Autodesk Inventor part; units mm, degrees
ref_plane "YZ Plane" through (0, 0, 0) normal (1, 0, 0) x (0, 1, 0)
ref_plane "XZ Plane" through (0, 0, 0) normal (0, 1, 0) x (-1, 0, 0)
ref_plane "XY Plane" through (0, 0, 0) normal (0, 0, 1) x (1, 0, 0)
sketch "スケッチ1" plane through (0, 0, 0) normal (0, 0, 1) x (1, 0, 0)
  circle A0 centre (0, 0) radius 7.5
  circle A1 centre (0, 0) radius 2
  dimension "d0" = 15
  dimension "d1" = 4
extrude "押し出し1" add sketch "スケッチ1" along normal blind 10 contours A1
extrude "押し出し2" add sketch "スケッチ1" against normal blind 15 contours A0 | A1
sketch "スケッチ2" plane through (0, 0, -15) normal (0, 0, -1) x (-1, 0, 0)
  circle A0 centre (0, 0) radius 7.5
hole "穴1" at (0, 0, -15) direction (0, 0, 1) diameter 3.3 depth 4 tip angle 118
properties part number "防振ゴム雄ねじ雌ねじm4スペーサー長さ15"
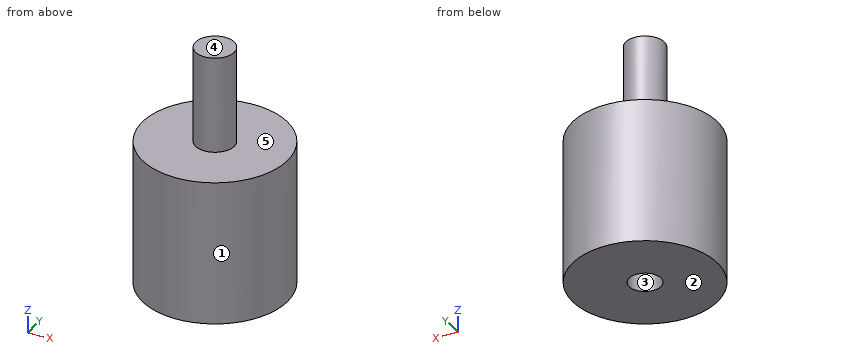
Work out the finished part from the listing and answer in its coordinate system (mm). Face numbers are marked on the shaded views. A direction names the side the tool comes from. Give positions to 0.01 mm unless a question says otherwise; leave off trailing zeros. Loops run counter-clockwise (first coordinate to the right, second up) from the corner with the lowest first, then second, coordinate; pieces in that order, holes last. Notation, with made-up numbers: (-25, -5.75) -> (27, -5.75) arc R16 cw to (27, 24.25) -> close; hole circle Ø4 at (68.5, 8.5). An arc over 180 degrees is marked (long way). Use a Markdown table: item, result. Add a question column.
1) The part is cut by section B-B, the plane z = -12. Determine the outline of the cut face in (x, y), plus the area to 3 significant figures.
2) The part is cut by section C-C, the plane x = 6.75. Determine the outline of the cut face in (y, z).
3) Each of these flat-tipped pins is pushed along its axis until it touches: P1, Ø1, axis at x = 0.5, y = 1, coming from the -Z side; P2, Ø2, axis at y = -1.5, z = 2, coming from the -X side; P3, Ø5, axis at x = 3.5, y = -3, coming from the +Z side. Where does it stop, or does it pass through?
4) The part is cut by section D-D, the plane y = -2.5. Determine the outline of the cut face in (x, z), plus the area to 3 significant figures.
5) Which of the six approach directions +Z, -Z, +X, -X, +Y, -Y give full straight-line access (tool end or side, diameter ignored) to the marked faces 4 and 5?
6) For a pull along X with two mould halves and no side action, classify the marked faces 1, 2 and 3 as +X half, -X half, draft (parallel to the pull), parting line (faces both ways), or undercut.
7) The part is cut by section A-A, the plane z = -6.25. Determine the outline of the cut face in (x, y).
8) Consider line 1 along Y through (x, z) = (0, -13.3); line 2 along Z through (x, y) = (-3.5, -4); line 3 along Y through (x, z) = (0.5, 8.5). Determine where each line is inside the solid, lowest interval first.
Reported:
| question | item | result |
|---|---|---|
| 1 | outline | circle Ø15 at (0, 0); hole circle Ø3.3 at (0, 0) |
| 1 | area | 168 mm^2 |
| 2 | outline | (-3.27, -15) -> (3.27, -15) -> (3.27, 0) -> (-3.27, 0) -> close |
| 3 | P1 | stops at z = -10.98 |
| 3 | P2 | stops at x = -1.94 |
| 3 | P3 | stops at z = 0 |
| 4 | outline | (-7.07, -15) -> (7.07, -15) -> (7.07, 0) -> (-7.07, 0) -> close |
| 4 | area | 212 mm^2 |
| 5 | face 4 | +Z, +X, -X, +Y, -Y |
| 5 | face 5 | +Z |
| 6 | face 1 | parting line |
| 6 | face 2 | draft |
| 6 | face 3 | undercut |
| 7 | outline | circle Ø15 at (0, 0) |
| 8 | line 1 | y = -7.5 to -1.65, 1.65 to 7.5 |
| 8 | line 2 | z = -15 to 0 |
| 8 | line 3 | y = -1.94 to 1.94 |
